Input: part model. Units: mm. Frame: model coordinates. Face numbers are marked on the shaded views. A direction names the side the tool comes from. Coordinates: 2 decimals unless noted, no trailing zeros. Loops run counter-clockwise (first coordinate to the right, second up) from the corner with the lowest first, then second, coordinate; pieces in that order, holes last.
(1) Section C-C, the plane x = 43. Return loops of the section in (y, z), then the cut area to 3 significant figures.
(2) Set-up query: the marked faces 4, 5 and 6. Return all of +Z, -Z, +X, -X, +Y, -Y with unobstructed straight access to the full face (end or side cutting, diameter ignored); none if empty.
(3) Line query: L1, parallel to Y at x = 39, z = -79.5; L2, parallel to X at y = 8, z = -136; L3, parallel to Y at x = 3.5, z = -97. Output: solid intervals per line, ascending.
(4) Section B-B, the plane y = 118. Return loops of the section in (x, z), then the cut area to 3 significant figures.
(5) Section D-D, the plane z = -95.5. Return loops of the section in (x, y).
(6) Contact query for flat-ended pins moving along their axis: P1, Ø10, axis at x = 7.5, y = -73, coming from the -Z side; P2, Ø15, axis at x = 27.5, z = -160.5, coming from the -Y side; P3, Ø7.5, axis at x = 25.4, z = -239.82, coming from the -Y side; P4, Ø3.5, axis at x = 25.4, z = -189.02, coming from the -Y side. Output: stop coordinate, or through.
(7) Section A-A, the plane x = 25.4. Return loops of the section in (y, z), then the cut area to 3 significant figures.
(8) Mould query, pull axis Z, two halves, no side actions, for the marked faces 1, 2 and 3. Classes: released by +Z, released by -Z, zero draft, split by the parting line, or undercut.
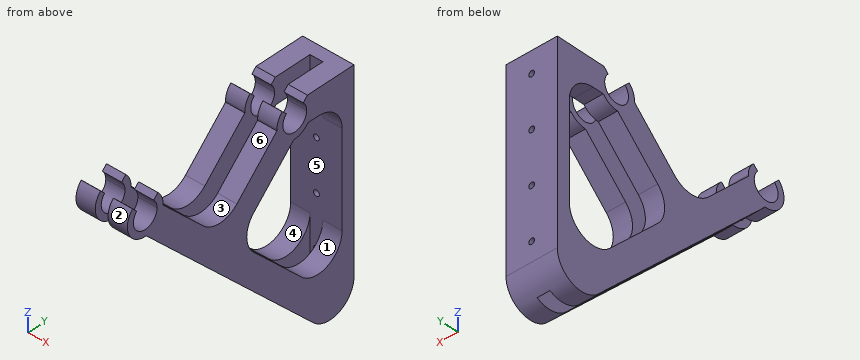
```python
from build123d import *

# Parameters (mm, degrees)
F1_DEPTH = 50.8
F3_W     = 12.7
F3_H     = 218.0215369846
F4_DEPTH = 254
F5_R     = 2.8575
F6_DEPTH = 12.701


with BuildPart() as f1:
    # F0 (on Right) → F1 (new body)
    with BuildSketch(Plane.YZ):
        with BuildLine():
            ThreePointArc((92.3909342397, -79.6909342397), (74.8308546487, -91.4242043026), (70.7106781187, -70.7106781187))
            ThreePointArc((70.7106781187, -70.7106781187), (65.8235712608, -75.2811893269), (60.6417499855, -79.5146411593))
            ThreePointArc((60.6417499855, -79.5146411593), (60.6460643138, -80.133008335), (60.6704465476, -80.7509096897))
            Line((60.6704465476, -80.7509096897), (17.9605122421, -123.4608439952))
            ThreePointArc((17.9605122421, -123.4608439952), (0, -130.900331753), (-17.9605122421, -123.4608439952))
            Line((-17.9605122421, -123.4608439952), (-60.6704465476, -80.7509096897))
            ThreePointArc((-60.6704465476, -80.7509096897), (-60.6460643138, -80.133008335), (-60.6417499855, -79.5146411593))
            ThreePointArc((-60.6417499855, -79.5146411593), (-65.8235712608, -75.2811893269), (-70.7106781187, -70.7106781187))
            ThreePointArc((-70.7106781187, -70.7106781187), (-67.9576641768, -74.8308546487), (-66.9909342397, -79.6909342397))
            ThreePointArc((-66.9909342397, -79.6909342397), (-84.5510138308, -91.4242043026), (-88.6711903608, -70.7106781187))
            Line((-88.6711903608, -70.7106781187), (-93.1613184213, -66.2205500581))
            ThreePointArc((-93.1613184213, -66.2205500581), (-97.0811254405, -87.4680641731), (-78.6309587898, -98.7114219318))
            Line((-78.6309587898, -98.7114219318), (99.4602185633, -276.8025992848))
            ThreePointArc((99.4602185633, -276.8025992848), (127.1408899875, -282.3086271685), (142.8207308054, -258.8420870427))
            Line((142.8207308054, -258.8420870427), (142.8207308054, -66.2205500581))
            Line((142.8207308054, -66.2205500581), (130.1207308054, -66.2205500581))
            Line((130.1207308054, -66.2205500581), (93.1613184213, -66.2205500581))
            Line((93.1613184213, -66.2205500581), (88.6711903608, -70.7106781187))
            ThreePointArc((88.6711903608, -70.7106781187), (91.4242043026, -74.8308546487), (92.3909342397, -79.6909342397))
        make_face()
        with BuildLine():
            ThreePointArc((78.6309587898, -98.7114219318), (87.0857697361, -96.9419835869), (93.8899658968, -91.6205500581))
            Line((93.8899658968, -91.6205500581), (104.7207308054, -91.6205500581))
            ThreePointArc((104.7207308054, -91.6205500581), (122.6812430475, -99.060037816), (130.1207308054, -117.0205500581))
            Line((130.1207308054, -117.0205500581), (130.1207308054, -210.2210625584))
            ThreePointArc((130.1207308054, -210.2210625584), (114.4408899875, -233.6876026842), (86.7602185633, -228.1815748006))
            Line((86.7602185633, -228.1815748006), (35.9210244843, -177.3423807216))
            ThreePointArc((35.9210244843, -177.3423807216), (28.4815367264, -159.3818684794), (35.9210244843, -141.4213562373))
            Line((35.9210244843, -141.4213562373), (78.6309587898, -98.7114219318))
        make_face(mode=Mode.SUBTRACT)
        with BuildLine():
            ThreePointArc((60.6417499855, -79.5146411593), (65.8235712608, -75.2811893269), (70.7106781187, -70.7106781187))
            Line((70.7106781187, -70.7106781187), (66.2205500581, -66.2205500581))
            ThreePointArc((66.2205500581, -66.2205500581), (62.1249501408, -72.3194552405), (60.6417499855, -79.5146411593))
        make_face()
        with BuildLine():
            Line((-66.2205500581, -66.2205500581), (-70.7106781187, -70.7106781187))
            ThreePointArc((-70.7106781187, -70.7106781187), (-65.8235712608, -75.2811893269), (-60.6417499855, -79.5146411593))
            ThreePointArc((-60.6417499855, -79.5146411593), (-62.1249501408, -72.3194552405), (-66.2205500581, -66.2205500581))
        make_face()
    extrude(amount=F1_DEPTH)

    # F3 (on offset) → F4 (cut, through all)
    with BuildSketch(Plane.XZ.offset(123.8792691946)):
        with Locations((25.4, -175.2313185504)):
            Rectangle(F3_W, F3_H)
    extrude(amount=-F4_DEPTH, mode=Mode.SUBTRACT)

    # F5 (on face) → F6 (cut, through all)
    with BuildSketch(Plane.XZ.offset(-130.1207308054)):
        with Locations((25.4, -138.2208063083)):
            Circle(F5_R)
        with Locations((25.4, -87.4208063083)):
            Circle(F5_R)
        with Locations((25.4, -239.8208063083)):
            Circle(F5_R)
        with Locations((25.4, -189.0208063083)):
            Circle(F5_R)
    extrude(amount=-F6_DEPTH, mode=Mode.SUBTRACT)


solid = f1.part
```
Report:
1. outline: (-93.16, -66.22) arc R19.05 ccw to (-78.63, -98.71) - (99.46, -276.8) arc R25.4 ccw to (142.82, -258.84) - (142.82, -66.22) - (93.16, -66.22) - (88.67, -70.71) arc R12.7 cw (long way) to (70.71, -70.71) - (66.22, -66.22) arc R19.05 ccw to (60.67, -80.75) - (17.96, -123.46) arc R25.4 cw to (-17.96, -123.46) - (-60.67, -80.75) arc R19.05 ccw to (-66.22, -66.22) - (-70.71, -70.71) arc R12.7 cw (long way) to (-88.67, -70.71) - close; hole (35.92, -177.34) - (86.76, -228.18) arc R25.4 ccw to (130.12, -210.22) - (130.12, -117.02) arc R25.4 ccw to (104.72, -91.62) - (93.89, -91.62) arc R19.05 cw to (78.63, -98.71) - (35.92, -141.42) arc R25.4 ccw to start
1. area: 14,500 mm2
2. face 4: +X, -X
2. face 5: none
2. face 6: +Z, +X, -X
3. L1: y = -98.74 to -92.39, -66.99 to -60.64, 60.64 to 66.99, 92.39 to 142.82
3. L2: x = 0 to 19.05, 31.75 to 50.8
3. L3: y = -87.65 to -44.42, 44.42 to 86.96, 120.35 to 142.82
4. outline: (0, -284.24) - (19.05, -284.24) - (19.05, -231.87) - (0, -231.87) - close; (0, -95.37) - (19.05, -95.37) - (19.05, -66.22) - (0, -66.22) - close; (31.75, -284.24) - (50.8, -284.24) - (50.8, -231.87) - (31.75, -231.87) - close; (31.75, -95.37) - (50.8, -95.37) - (50.8, -66.22) - (31.75, -66.22) - close
4. area: 3,110 mm2
5. outline: (0, -90.32) - (19.05, -90.32) - (19.05, -45.92) - (0, -45.92) - close; (0, 45.92) - (19.05, 45.92) - (19.05, 89.65) - (0, 89.65) - close; (0, 118.21) - (19.05, 118.21) - (19.05, 130.12) - (31.75, 130.12) - (31.75, 118.21) - (50.8, 118.21) - (50.8, 142.82) - (0, 142.82) - close; (31.75, -90.32) - (50.8, -90.32) - (50.8, -45.92) - (31.75, -45.92) - close; (31.75, 45.92) - (50.8, 45.92) - (50.8, 89.65) - (31.75, 89.65) - close
6. P1: stops at z = -109.34
6. P2: stops at y = -23.02
6. P3: stops at y = 130.12
6. P4: passes through
7. outline: (130.12, -280.84) arc R25.4 ccw to (142.82, -258.84) - (142.82, -242.68) - (130.12, -242.68) - close; (130.12, -236.96) - (142.82, -236.96) - (142.82, -191.88) - (130.12, -191.88) - close; (130.12, -186.16) - (142.82, -186.16) - (142.82, -141.08) - (130.12, -141.08) - close; (130.12, -135.36) - (142.82, -135.36) - (142.82, -90.28) - (130.12, -90.28) - close; (130.12, -84.56) - (142.82, -84.56) - (142.82, -66.22) - (130.12, -66.22) - close
7. area: 2,350 mm2
8. face 1: undercut
8. face 2: split by the parting line
8. face 3: released by +Z
